Could you check a few things on this model? Use its own coordinates, in mm. Face numbers are marked on the shaded views. A direction names the side the tool comes from. Coordinates: 2 decimals unless noted, no trailing zeros. Write each loop counter-clockwise with the first axis right and the second up, starting at its lowest first coordinate (ties: lowest second). Pieces come first, ordered by that corner, then holes. Notation, with made-up numbers: (27, 39.25) - (40, 39.25) arc R14 cw to (40, 64.25) - close; hole circle Ø11 at (86, 49.5). An arc over 180 degrees is marked (long way). Write item = value, one per line. Start each with the question number.
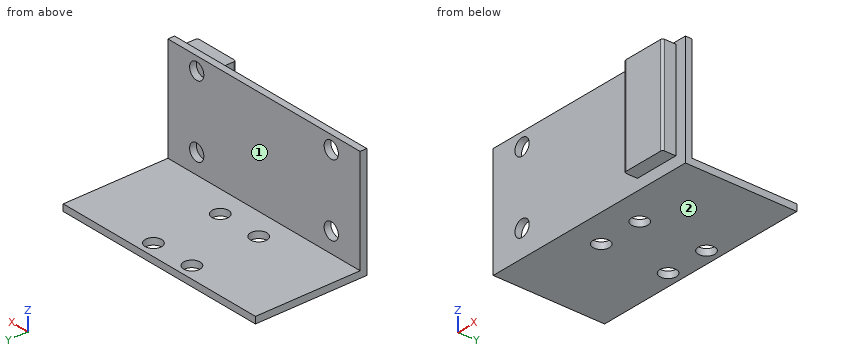
```python
from build123d import *

# Parameters (mm, degrees)
SKETCH1_W           = 50
SKETCH1_H           = 25
BOSS_EXTRUDE1_DEPTH = 1.5
SKETCH3_W           = 50
SKETCH3_H           = 1.5
BOSS_EXTRUDE2_DEPTH = 23.5
SKETCH4_R           = 1.85
CUT_EXTRUDE1_DEPTH  = 23
SKETCH5_R           = 1.85
CUT_EXTRUDE2_DEPTH  = 23
SKETCH6_W           = 10
SKETCH6_H           = 22
BOSS_EXTRUDE3_DEPTH = 3
FILLET1_R           = 0.5


with BuildPart() as part:
    # Sketch1 → Boss-Extrude1 (new body)
    with BuildSketch(Plane(origin=(0, 0, 0), x_dir=(1, 0, 0), z_dir=(0, 1, 0))):
        with Locations((25, 12.5)):
            Rectangle(SKETCH1_W, SKETCH1_H)
    extrude(amount=BOSS_EXTRUDE1_DEPTH)

    # Sketch3 → Boss-Extrude2 (add)
    with BuildSketch(Plane(origin=(0, 1.5, 0), x_dir=(1, 0, 0), z_dir=(0, 1, 0))):
        with Locations((25, 24.25)):
            Rectangle(SKETCH3_W, SKETCH3_H)
    extrude(amount=BOSS_EXTRUDE2_DEPTH)

    # Sketch4 → Cut-Extrude1 (cut)
    with BuildSketch(Plane.XY.offset(-23.5)):
        with Locations((20, 22)):
            Circle(SKETCH4_R)
        with Locations((30, 22)):
            Circle(SKETCH4_R)
        with Locations((30, 7)):
            Circle(SKETCH4_R)
        with Locations((20, 7)):
            Circle(SKETCH4_R)
    extrude(amount=-CUT_EXTRUDE1_DEPTH, mode=Mode.SUBTRACT)

    # Sketch5 → Cut-Extrude2 (cut)
    with BuildSketch(Plane(origin=(0, 1.5, 0), x_dir=(1, 0, 0), z_dir=(0, 1, 0))):
        with Locations((7.5, 3)):
            Circle(SKETCH5_R)
        with Locations((7.5, 19)):
            Circle(SKETCH5_R)
        with Locations((42.5, 3)):
            Circle(SKETCH5_R)
        with Locations((42.5, 19)):
            Circle(SKETCH5_R)
    extrude(amount=-CUT_EXTRUDE2_DEPTH, mode=Mode.SUBTRACT)

    # Sketch6 → Boss-Extrude3 (add)
    with BuildSketch(Plane.XZ):
        with Locations((42.5, -11.5)):
            Rectangle(SKETCH6_W, SKETCH6_H)
    extrude(amount=BOSS_EXTRUDE3_DEPTH)

    # Fillet1
    fillet1_edges = [part.edges().sort_by_distance(p)[0] for p in [
        (47.5, -3, -11.5),
        (37.5, -3, -11.5),
    ]]
    fillet(fillet1_edges, radius=FILLET1_R)


solid = part.part
```
1) Suppose I cut it at D-D on x = 42.5. Please give me the cut outline in (y, z).
2) If I drill on probe 1 along X at (y, z) = (0.75, -19); probe 2 along Y at (x, z) = (20, -24.05); probe 3 along Z at (x, y) = (7.5, 0.75), over which ranges is the centre line in solid material (lowest first)? Write a range as [from, to].
3) Suppose I cut it at C-C on x = 20. Please give me the cut outline in (y, z).
4) Suppose I cut it at A-A on z = -3. Please give me the cut outline in (x, y), plus the area to 3 significant figures.
5) Suppose I cut it at B-B on y = 7. Please give me the cut outline in (x, z), plus the area to 3 significant figures.
6) For P1, Ø8, axis at x = 22, y = 9.5, coming from the +Z side; P2, Ø0.8, axis at y = -1.5, z = -8, coming from the -X side; P3, Ø3, axis at x = 43, z = -2.5, coming from the +Y side, each with a flat end and sliding along its axis, tell me the tip position at first contact or that it passes through.
7) Which directions (+Z, -Z, +X, -X, +Y, -Y) give clear straight access to the entire face, cutting with the end or side of a thin tool? Please do the marked faces 1 and 2.
Reply:
q1.outline = (-3, -22.5) - (0, -22.5) - (0, -25) - (25, -25) - (25, -23.5) - (1.5, -23.5) - (1.5, -20.85) - (0, -20.85) - (0, -17.15) - (1.5, -17.15) - (1.5, -4.85) - (0, -4.85) - (0, -1.15) - (1.5, -1.15) - (1.5, 0) - (0, 0) - (0, -0.5) - (-3, -0.5) - close
q2.probe_1 = [0, 5.65], [9.35, 40.65], [44.35, 50]
q2.probe_2 = [0, 5.15], [8.85, 20.15], [23.85, 25]
q2.probe_3 = [-25, -20.85], [-17.15, -4.85], [-1.15, 0]
q3.outline = (0, -25) - (5.15, -25) - (5.15, -23.5) - (1.5, -23.5) - (1.5, 0) - (0, 0) - close; (8.85, -25) - (20.15, -25) - (20.15, -23.5) - (8.85, -23.5) - close; (23.85, -25) - (25, -25) - (25, -23.5) - (23.85, -23.5) - close
q4.outline = (0, 0) - (5.65, 0) - (5.65, 1.5) - (0, 1.5) - close; (9.35, 0) - (37.5, 0) - (37.5, -2.5) arc R0.5 ccw to (38, -3) - (47, -3) arc R0.5 ccw to (47.5, -2.5) - (47.5, 0) - (50, 0) - (50, 1.5) - (44.35, 1.5) - (44.35, 0) - (40.65, 0) - (40.65, 1.5) - (9.35, 1.5) - close
q4.area = 93.8 mm^2
q5.outline = (0, -25) - (18.15, -25) - (18.15, -23.5) - (0, -23.5) - close; (21.85, -25) - (28.15, -25) - (28.15, -23.5) - (21.85, -23.5) - close; (31.85, -25) - (50, -25) - (50, -23.5) - (31.85, -23.5) - close
q5.area = 63.9 mm^2
q6.P1 = -23.5
q6.P2 = 37.5
q6.P3 = 1.5
q7.face_1 = +Z, +X, -X, +Y
q7.face_2 = -Z, +X, -X, +Y, -Y
